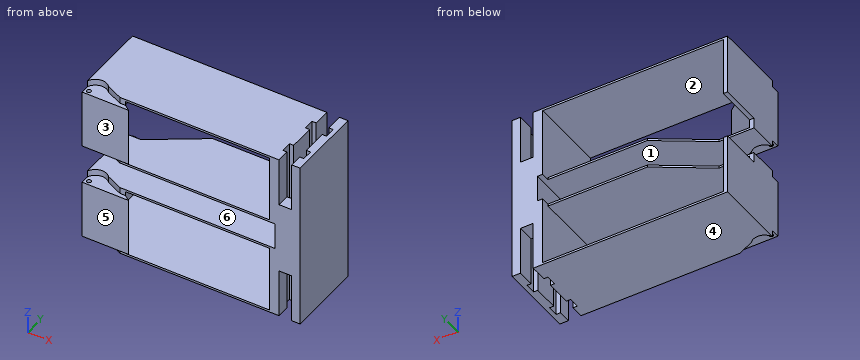
```python
from build123d import *

# Parameters (mm, degrees)
SKETCH2_W            = 89.5
SKETCH2_H            = 33.7
BOSS_EXTRUDE1_DEPTH  = 38
SKETCH3_W            = 85.5
SKETCH3_H            = 31.7
CUT_EXTRUDE1_DEPTH   = 38
BOSS_EXTRUDE2_DEPTH  = 31.7
SKETCH5_W            = 33.7
SKETCH5_H            = 38
BOSS_EXTRUDE3_DEPTH  = 2.5
SKETCH6_W            = 2
SKETCH6_H            = 38
BOSS_EXTRUDE4_DEPTH  = 6.3
SKETCH7_W            = 34
SKETCH7_H            = 38
BOSS_EXTRUDE5_DEPTH  = 10
SKETCH8_W            = 4
SKETCH8_H            = 38
BOSS_EXTRUDE6_DEPTH  = 23
CUT_EXTRUDE2_START   = -32.7
SKETCH9_W            = 10
SKETCH9_H            = 5
CUT_EXTRUDE2_DEPTH   = 32.7
SKETCH11_W           = 80
SKETCH11_H           = 2
CUT_EXTRUDE3_DEPTH   = 80
CUT_EXTRUDE4_DEPTH   = 3
MIRROR4_COPY_1_DEPTH = 3
CUT_EXTRUDE5_START   = -74
SKETCH13_R           = 1
CUT_EXTRUDE5_DEPTH   = 74
SKETCH15_W           = 47
SKETCH15_H           = 1
CUT_EXTRUDE6_DEPTH   = 4
SKETCH16_W           = 40.5
SKETCH16_H           = 2
CUT_EXTRUDE7_DEPTH   = 19.9
SKETCH17_W           = 2
SKETCH17_H           = 19.9
CUT_EXTRUDE8_DEPTH   = 3
BOSS_EXTRUDE7_START  = -1
BOSS_EXTRUDE7_DEPTH  = 1


with BuildPart() as part:
    # Sketch2 → Boss-Extrude1 (new body)
    with BuildSketch(Plane(origin=(0, 0, 0), x_dir=(1, 0, 0), z_dir=(0, 1, 0))):
        Rectangle(SKETCH2_W, SKETCH2_H)
    extrude(amount=BOSS_EXTRUDE1_DEPTH)

    # Sketch3 → Cut-Extrude1 (cut)
    with BuildSketch(Plane(origin=(0, 38, 0), x_dir=(1, 0, 0), z_dir=(0, 1, 0))):
        Rectangle(SKETCH3_W, SKETCH3_H)
    extrude(amount=-CUT_EXTRUDE1_DEPTH, mode=Mode.SUBTRACT)

    # Sketch4 → Boss-Extrude2 (add)
    with BuildSketch(Plane.XY.offset(-15.85)):
        Polygon((-42.75, 0), (-42.75, 15), (-22.75, 0), align=None)
    extrude(amount=BOSS_EXTRUDE2_DEPTH)

    # Sketch5 → Boss-Extrude3 (add)
    with BuildSketch(Plane(origin=(44.75, 0, 0), x_dir=(0, 0, -1), z_dir=(1, 0, 0))):
        with Locations((0, 19)):
            Rectangle(SKETCH5_W, SKETCH5_H)
    extrude(amount=BOSS_EXTRUDE3_DEPTH)

    # Sketch6 → Boss-Extrude4 (add)
    with BuildSketch(Plane(origin=(0, 0, -16.85), x_dir=(-1, 0, 0), z_dir=(0, 0, -1))):
        with Locations((-46.25, 19)):
            Rectangle(SKETCH6_W, SKETCH6_H)
    extrude(amount=BOSS_EXTRUDE4_DEPTH)

    # Mirror1: part across plane


with BuildPart() as part_1:
    add(part.part)
    add(part.part.mirror(Plane(origin=(0, 0, -23.15), x_dir=(1, 0, 0), z_dir=(0, 0, -1))))

    # Sketch7 → Boss-Extrude5 (add)
    with BuildSketch(Plane(origin=(47.25, 0, 0), x_dir=(0, 0, -1), z_dir=(1, 0, 0))):
        with Locations((23.15, 19)):
            Rectangle(SKETCH7_W, SKETCH7_H)
    extrude(amount=BOSS_EXTRUDE5_DEPTH)

    # Sketch8 → Boss-Extrude6 (add)
    with BuildSketch(Plane.XY.offset(-6.15)):
        with Locations((55.25, 19)):
            Rectangle(SKETCH8_W, SKETCH8_H)
    boss_extrude6 = extrude(amount=BOSS_EXTRUDE6_DEPTH)

    # Sketch9 → Cut-Extrude2 (cut)
    with BuildSketch(Plane.XY.offset(16.85).offset(CUT_EXTRUDE2_START)):
        with Locations((50.25, 27.5)):
            Rectangle(SKETCH9_W, SKETCH9_H)
        with Locations((50.25, 10.5)):
            Rectangle(SKETCH9_W, SKETCH9_H)
    cut_extrude2 = extrude(amount=CUT_EXTRUDE2_DEPTH, mode=Mode.SUBTRACT)

    # Mirror2: Boss-Extrude6, Cut-Extrude2 across plane
    add(boss_extrude6.mirror(Plane(origin=(0, 0, -23.15), x_dir=(1, 0, 0), z_dir=(0, 0, -1))))
    add(cut_extrude2.mirror(Plane(origin=(0, 0, -23.15), x_dir=(1, 0, 0), z_dir=(0, 0, -1))), mode=Mode.SUBTRACT)

    # Sketch11 → Cut-Extrude3 (cut)
    with BuildSketch(Plane(origin=(57.25, 0, 0), x_dir=(0, 0, -1), z_dir=(1, 0, 0))):
        with Locations((23.15, 1)):
            Rectangle(SKETCH11_W, SKETCH11_H)
    extrude(amount=-CUT_EXTRUDE3_DEPTH, mode=Mode.SUBTRACT)

    # Sketch12 → Cut-Extrude4 (cut)
    with BuildSketch(Plane.XY.offset(16.85)):
        with BuildLine():
            Line((-22.75, 2), (-34.364835193, 2))
            ThreePointArc((-34.364835193, 2), (-40.768375168, 7.287996976), (-44.75, 0))
            Line((-44.75, 0), (-22.75, 0))
            Line((-22.75, 0), (-22.75, 2))
        make_face()
    cut_extrude4 = extrude(amount=-CUT_EXTRUDE4_DEPTH, mode=Mode.SUBTRACT)

    # Mirror3: Cut-Extrude4 across plane
    add(cut_extrude4.mirror(Plane.XY), mode=Mode.SUBTRACT)

    # Mirror4: Cut-Extrude4 across plane
    add(cut_extrude4.mirror(Plane(origin=(0, 0, -23.15), x_dir=(1, 0, 0), z_dir=(0, 0, -1))), mode=Mode.SUBTRACT)

    # Mirror4 copy 1 sketch → Mirror4 copy 1 (cut)
    with BuildSketch(Plane.XY.offset(-29.45)):
        with BuildLine():
            Line((-22.75, 2), (-34.364835193, 2))
            ThreePointArc((-34.364835193, 2), (-40.768375168, 7.287996976), (-44.75, 0))
            Line((-44.75, 0), (-22.75, 0))
            Line((-22.75, 0), (-22.75, 2))
        make_face()
    extrude(amount=-MIRROR4_COPY_1_DEPTH, mode=Mode.SUBTRACT)

    # Sketch13 → Cut-Extrude5 (cut)
    with BuildSketch(Plane.XY.offset(13.85).offset(CUT_EXTRUDE5_START)):
        with Locations((-42.75, 2)):
            Circle(SKETCH13_R)
    extrude(amount=CUT_EXTRUDE5_DEPTH, mode=Mode.SUBTRACT)

    # Chamfer1
    # the kernel refuses this chamfer: 10 mm, written as the material it takes off along each edge
    with BuildSketch(Plane(origin=(-34.364835193, 2, 33.530669666), x_dir=(-0.4115208033655663, 0.9114003666870882, 0), z_dir=(0, 0, -1))) as chamfer1_piece_1:
        with BuildLine():
            Line((4.024103798, 0), (-2.897424879, 6.010331734))
            Line((-2.897424879, 6.010331734), (-3.079704953, 5.928027573))
            ThreePointArc((-3.079704953, 5.928027573), (-1.554736759, 2.957293148), (-0.182280073, -0.082304161))
            Line((-0.182280073, -0.082304161), (0.082304161, -0.182280073))
            ThreePointArc((0.082304161, -0.182280073), (2.000716354, 0.27264804), (3.968173362, -0.192020276))
            Line((3.968173362, -0.192020276), (4.024103798, 0))
        make_face()
    extrude(amount=19.680669666, mode=Mode.SUBTRACT)

    # Chamfer2
    # the kernel refuses this chamfer: 10 mm, written as the material it takes off along each edge
    with BuildSketch(Plane(origin=(-34.364835193, 2, -33.530669666), x_dir=(0.9996854583228201, -0.025079561756403367, 0), z_dir=(0, 0, 1))) as chamfer2_piece_1_section:
        with BuildLine():
            Line((6.304869905, 0.158173126), (-1.380064624, 3.466711132))
            ThreePointArc((-1.380064624, 3.466711132), (-0.439598609, 1.999919309), (0, 0))
            Line((0, 0), (6.304869905, 0.158173126))
        make_face()
    chamfer2_piece_1 = extrude(amount=19.680669666, mode=Mode.PRIVATE)
    chamfer2_piece_1 = split(chamfer2_piece_1, bisect_by=Plane(origin=(-32.514060805, 3.115216655, -29.45), z_dir=(0, 0, 1)), keep=Keep.TOP, mode=Mode.PRIVATE)
    add(chamfer2_piece_1, mode=Mode.SUBTRACT)

    # Chamfer3
    # the kernel refuses this chamfer: 10 mm, written as the material it takes off along each edge
    with BuildSketch(Plane(origin=(-34.364835193, 2, -12.769330334), x_dir=(-0.4115208033655663, 0.9114003666870882, 0), z_dir=(0, 0, -1))) as chamfer3_piece_1_section:
        with BuildLine():
            Line((4.024103798, 0), (-2.897424879, 6.010331734))
            Line((-2.897424879, 6.010331734), (-3.079704953, 5.928027573))
            ThreePointArc((-3.079704953, 5.928027573), (-1.554736759, 2.957293148), (-0.182280073, -0.082304161))
            Line((-0.182280073, -0.082304161), (0.082304161, -0.182280073))
            ThreePointArc((0.082304161, -0.182280073), (2.000716354, 0.27264804), (3.968173362, -0.192020276))
            Line((3.968173362, -0.192020276), (4.024103798, 0))
        make_face()
    chamfer3_piece_1 = extrude(amount=19.680669666, mode=Mode.PRIVATE)
    chamfer3_piece_1 = split(chamfer3_piece_1, bisect_by=Plane(origin=(-32.482113907, 3.03712607, -13.85), z_dir=(0, 0, -1)), keep=Keep.TOP, mode=Mode.PRIVATE)
    add(chamfer3_piece_1, mode=Mode.SUBTRACT)

    # Chamfer4
    # the kernel refuses this chamfer: 10 mm, written as the material it takes off along each edge
    with BuildSketch(Plane(origin=(-34.364835193, 2, -79.830669666), x_dir=(0.9996854583228201, -0.025079561756403367, 0), z_dir=(0, 0, 1))) as chamfer4_piece_1:
        with BuildLine():
            Line((6.672267866, 0), (-1.747462586, 3.624884258))
            Line((-1.747462586, 3.624884258), (-1.896145364, 3.491117927))
            ThreePointArc((-1.896145364, 3.491117927), (-0.623209418, 1.920628258), (-0.199937092, -0.005015912))
            Line((-0.199937092, -0.005015912), (0.005015912, -0.199937092))
            ThreePointArc((0.005015912, -0.199937092), (3.339051469, -0.116294632), (6.677283779, -0.199937092))
            Line((6.677283779, -0.199937092), (6.672267866, 0))
        make_face()
    extrude(amount=19.680669666, mode=Mode.SUBTRACT)

    # Sketch15 → Cut-Extrude6 (cut)
    with BuildSketch(Plane(origin=(0, 38, 0), x_dir=(1, 0, 0), z_dir=(0, 1, 0))):
        with Locations((19.25, 16.35)):
            Rectangle(SKETCH15_W, SKETCH15_H)
    cut_extrude6 = extrude(amount=-CUT_EXTRUDE6_DEPTH, mode=Mode.SUBTRACT)

    # Sketch16 → Cut-Extrude7 (cut)
    with BuildSketch(Plane(origin=(0, 38, 0), x_dir=(1, 0, 0), z_dir=(0, 1, 0))):
        with Locations((-24.5, 15.85)):
            Rectangle(SKETCH16_W, SKETCH16_H)
    cut_extrude7 = extrude(amount=-CUT_EXTRUDE7_DEPTH, mode=Mode.SUBTRACT)

    # Sketch17 → Cut-Extrude8 (cut)
    with BuildSketch(Plane(origin=(0, 0, -14.85), x_dir=(-1, 0, 0), z_dir=(0, 0, -1))):
        with Locations((43.75, 28.05)):
            Rectangle(SKETCH17_W, SKETCH17_H)
    cut_extrude8 = extrude(amount=-CUT_EXTRUDE8_DEPTH, mode=Mode.SUBTRACT)

    # Sketch18 → Boss-Extrude7 (add)
    with BuildSketch(Plane.XY.offset(-15.85).offset(BOSS_EXTRUDE7_START)):
        Polygon((-4.25, 18.1), (-4.25, 34), (-28.25, 18.1), align=None)
    boss_extrude7 = extrude(amount=BOSS_EXTRUDE7_DEPTH)

    # Mirror5: Cut-Extrude6, Cut-Extrude7, Cut-Extrude8, Boss-Extrude7 across plane
    add(cut_extrude6.mirror(Plane(origin=(0, 0, -23.15), x_dir=(1, 0, 0), z_dir=(0, 0, -1))), mode=Mode.SUBTRACT)
    add(cut_extrude7.mirror(Plane(origin=(0, 0, -23.15), x_dir=(1, 0, 0), z_dir=(0, 0, -1))), mode=Mode.SUBTRACT)
    add(cut_extrude8.mirror(Plane(origin=(0, 0, -23.15), x_dir=(1, 0, 0), z_dir=(0, 0, -1))), mode=Mode.SUBTRACT)
    add(boss_extrude7.mirror(Plane(origin=(0, 0, -23.15), x_dir=(1, 0, 0), z_dir=(0, 0, -1))))


solid = part_1.part
```
Verification items for the finished model (mm, model axes). Face numbers are marked on the shaded views. A direction names the side the tool comes from. Coordinates: 2 decimals unless noted, no trailing zeros. Loops run counter-clockwise (first coordinate to the right, second up) from the corner with the lowest first, then second, coordinate; pieces in that order, holes last. Notation, with made-up numbers: (-25.75, 23) -> (6.25, 23) arc R32 ccw to (6.25, 57) -> close; hole circle Ø4 at (25, -17). An arc over 180 degrees is marked (long way). Answer in a Markdown table with one row per item. Add a question column.
1. Material ranges on probe 1 along X at (y, z) = (23.5, -5); probe 2 along Z at (x, y) = (14.5, 36.5); probe 3 along Z at (x, y) = (19, 17), recorded low to high. Write a range as [from, to].
2. Depth check by flat-ended pin: P1, Ø1.5, axis at x = -38.5, z = -13, coming from the +Y side (3 decimals); P2, Ø5, axis at x = 34, z = -26.5, coming from the +Y side; P3, Ø11, axis at x = 50.5, z = -5.5, coming from the -Y side; P4, Ø2.5, axis at x = 49, y = 9.5, coming from the +Z side. Enter the tip coordinate at first touch or a pass-through.
3. Section check D-D, the plane x = -12.5. Enter the section's corners in (y, z), then the cut area to 3 significant figures.
4. Section check A-A, the plane z = -48. Give the number of separate pieces and of enclosed holes in the cut face, then the cut area to 3 significant figures.
5. Section check C-C, the plane x = -34.5. Enter the section's corners in (y, z).
6. Section check B-B, the plane x = 4.5. Enter the section's corners in (y, z).
7. Access from +Z, -Z, +X, -X, +Y, -Y to the whole of each face (thin tool, end or side, straight path). Record for the marked faces 1, 2 and 3.
8. Draft check along Z on the marked faces 4, 5 and 6. Enter one of: +Z half, -Z half, draft (parallel to the pull), parting line (faces both ways), or undercut.
Derived:
| question | item | result |
|---|---|---|
| 1 | probe 1 | x = [-44.75, -42.75], [42.75, 47.25], [53.25, 57.25] |
| 1 | probe 2 | z = [-63.15, -62.15], [15.85, 16.85] |
| 1 | probe 3 | z = [-63.15, -62.15], [-30.45, -29.45], [-16.85, -15.85], [15.85, 16.85] |
| 2 | P1 | stops at y = 12.375 |
| 2 | P2 | passes through |
| 2 | P3 | stops at y = 2 |
| 2 | P4 | stops at z = -15.85 |
| 3 | outline | (2, -63.15) -> (38, -63.15) -> (38, -62.15) -> (2, -62.15) -> close; (2, -30.45) -> (28.53, -30.45) -> (28.53, -29.45) -> (2, -29.45) -> close; (2, -16.85) -> (28.53, -16.85) -> (28.53, -15.85) -> (2, -15.85) -> close; (2, 15.85) -> (38, 15.85) -> (38, 16.85) -> (2, 16.85) -> close |
| 3 | area | 125 mm² |
| 4 | separate pieces | 3 |
| 4 | enclosed holes | 1 |
| 4 | area | 489 mm² |
| 5 | outline | (0, -60.15) -> (4.97, -60.15) -> (4.97, -63.15) -> (38, -63.15) -> (38, -62.15) -> (8.81, -62.15) -> (8.81, -30.45) -> (18.1, -30.45) -> (18.1, -29.45) -> (4.97, -29.45) -> (4.97, -32.45) -> (0, -32.45) -> close; (0, -13.85) -> (4.97, -13.85) -> (4.97, -16.85) -> (18.1, -16.85) -> (18.1, -15.85) -> (8.81, -15.85) -> (8.81, 15.85) -> (38, 15.85) -> (38, 16.85) -> (4.97, 16.85) -> (4.97, 13.85) -> (0, 13.85) -> close |
| 6 | outline | (2, -63.15) -> (38, -63.15) -> (38, -62.15) -> (2, -62.15) -> close; (2, -30.45) -> (34, -30.45) -> (34, -29.45) -> (2, -29.45) -> close; (2, -16.85) -> (34, -16.85) -> (34, -15.85) -> (2, -15.85) -> close; (2, 15.85) -> (38, 15.85) -> (38, 16.85) -> (2, 16.85) -> close |
| 7 | face 1 | -X, +Y, -Y |
| 7 | face 2 | +Y |
| 7 | face 3 | +Z, -Z, +X, -X, -Y |
| 8 | face 4 | -Z half |
| 8 | face 5 | draft |
| 8 | face 6 | undercut |
